Read the model definition and answer for the solid it produces. Units are mm, in the model's axes. Face numbers are marked on the shaded views. A direction names the side the tool comes from. Give positions to 0.01 mm unless a question says otherwise; leave off trailing zeros. Write each loop counter-clockwise with the first axis right and the second up, starting at its lowest first coordinate (ties: lowest second). Pieces come first, ordered by that corner, then holes. Notation, with made-up numbers: (-13.75, 83.5) - (0.25, 83.5) arc R33 ccw to (0.25, 117.5) - close; hole circle Ø3 at (-20.5, 21.25). An arc over 180 degrees is marked (long way). Answer as CSV lines item,"result".
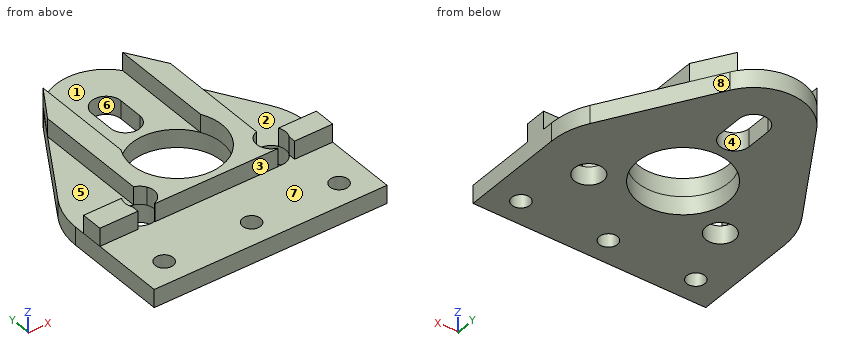
```python
from build123d import *

# Parameters (mm, degrees)
F0_R     = 2.5
F0_R_2   = 4
F0_R_3   = 12.5
F1_DEPTH = 5
F3_DEPTH = 5


# Not quite as in the source:
# - after a boolean that leaves OpenCascade's solid faulty, fix() repairs it


with BuildPart() as f1:
    # F0 (on Top) → F1 (new body)
    with BuildSketch(Plane.XY):
        with BuildLine():
            Line((-32.1865334795, -5.601415029), (-32.1865334795, -34.5))
            Line((-32.1865334795, -34.5), (32.1865334795, -34.5))
            Line((32.1865334795, -34.5), (32.1865334795, -5.601415029))
            ThreePointArc((32.1865334795, -5.601415029), (31.4454600423, -0.2075529944), (29.2771587146, 4.7865842524))
            Line((29.2771587146, 4.7865842524), (11.9634376646, 33.271599497))
            ThreePointArc((11.9634376646, 33.271599497), (0, 40), (-11.9634376646, 33.271599497))
            Line((-11.9634376646, 33.271599497), (-29.2771587146, 4.7865842524))
            ThreePointArc((-29.2771587146, 4.7865842524), (-31.4454600423, -0.2075529944), (-32.1865334795, -5.601415029))
        make_face()
        with Locations((-24.1865334795, -27.5)):
            Circle(F0_R, mode=Mode.SUBTRACT)
        with Locations((-18.1865334795, -10.5)):
            Circle(F0_R_2, mode=Mode.SUBTRACT)
        with Locations((0, -27.5)):
            Circle(F0_R, mode=Mode.SUBTRACT)
        with Locations((24.1865334795, -27.5)):
            Circle(F0_R, mode=Mode.SUBTRACT)
        Circle(F0_R_3, mode=Mode.SUBTRACT)
        with Locations((18.1865334795, -10.5)):
            Circle(F0_R_2, mode=Mode.SUBTRACT)
        with BuildLine():
            Line((-4, 21), (-4, 26))
            ThreePointArc((-4, 26), (0, 30), (4, 26))
            Line((4, 26), (4, 21))
            Line((4, 21), (4, 19))
            ThreePointArc((4, 19), (0, 15), (-4, 19))
            Line((-4, 19), (-4, 21))
        make_face(mode=Mode.SUBTRACT)
    extrude(amount=F1_DEPTH)

    # F2 (on face) → F3 (join)
    with BuildSketch(Plane.XY.offset(5)):
        with BuildLine():
            Line((-32.1865334795, -8.5), (-32.1865334795, -14.5))
            Line((-32.1865334795, -14.5), (-21.6506350946, -14.5))
            Line((-21.6506350946, -14.5), (-21.6506350946, -12.5))
            ThreePointArc((-21.6506350946, -12.5), (-22.1865334795, -10.5), (-21.6506350946, -8.5))
            Line((-21.6506350946, -8.5), (-32.1865334795, -8.5))
        make_face()
        with BuildLine():
            Line((21.6506350946, -14.5), (32.1865334795, -14.5))
            Line((32.1865334795, -14.5), (32.1865334795, -8.5))
            Line((32.1865334795, -8.5), (21.6506350946, -8.5))
            ThreePointArc((21.6506350946, -8.5), (22.1865334795, -10.5), (21.6506350946, -12.5))
            Line((21.6506350946, -12.5), (21.6506350946, -14.5))
        make_face()
        with BuildLine():
            ThreePointArc((17, -14.3199657462), (14.4616036791, -11.9577029816), (14.7224318643, -8.5))
            ThreePointArc((14.7224318643, -8.5), (15.6895011358, -7.3751272866), (17, -6.6800342538))
            Line((17, -6.6800342538), (17, 24.9853071114))
            Line((17, 24.9853071114), (11, 34.6602540378))
            Line((11, 34.6602540378), (11, 5.9371710435))
            ThreePointArc((11, 5.9371710435), (0, -12.5), (-11, 5.9371710435))
            Line((-11, 5.9371710435), (-11, 34.6602540378))
            Line((-11, 34.6602540378), (-17, 24.9853071114))
            Line((-17, 24.9853071114), (-17, -6.6800342538))
            ThreePointArc((-17, -6.6800342538), (-15.6895011358, -7.3751272866), (-14.7224318643, -8.5))
            ThreePointArc((-14.7224318643, -8.5), (-14.4616036791, -11.9577029816), (-17, -14.3199657462))
            Line((-17, -14.3199657462), (-17, -14.5))
            Line((-17, -14.5), (17, -14.5))
            Line((17, -14.5), (17, -14.3199657462))
        make_face()
    extrude(amount=F3_DEPTH)

    add(f1.part.fix(), mode=Mode.REPLACE)


solid = f1.part
```
(1) A cutting plane is placed at D-D (y = 18). Write down the section's boundary in (x, z), and give its area (3 significant figures).
Worked out:
outline,"(-21.25, 0) - (-3.87, 0) - (-3.87, 5) - (-11, 5) - (-11, 10) - (-17, 10) - (-17, 5) - (-21.25, 5) - close; (3.87, 0) - (21.25, 0) - (21.25, 5) - (17, 5) - (17, 10) - (11, 10) - (11, 5) - (3.87, 5) - close"
area,"234 mm^2"
(2) A cutting plane is placed at A-A (x = 0). Write down the section's boundary in (y, z), and give its area (4 significant figures).
Worked out:
outline,"(-34.5, 0) - (-30, 0) - (-30, 5) - (-34.5, 5) - close; (-25, 0) - (-12.5, 0) - (-12.5, 10) - (-14.5, 10) - (-14.5, 5) - (-25, 5) - close; (12.5, 0) - (15, 0) - (15, 5) - (12.5, 5) - close; (30, 0) - (40, 0) - (40, 5) - (30, 5) - close"
area,"157.5 mm^2"
(3) Each of these flat-tipped pins is pushed along its axis until it touches: P1, Ø6, axis at x = -24.5, z = 8.5, coming from the -Y side; P2, Ø2.5, axis at y = 2.5, z = 6.5, coming from the -X side; P3, Ø5.5, axis at y = 21.5, z = 3, coming from the -X side; P4, Ø1.8, axis at x = -15.5, y = 30, coming from the +Z side. Where does it stop, or does it pass through?
Worked out:
P1,"stops at y = -14.5"
P2,"stops at x = -17"
P3,"stops at x = -20.79"
P4,"passes through"
(4) The mould has two halves that part along Y. Classify the marked faces 6, 7 and 8: +Y half, -Y half, draft (parallel to the pull), parting line (faces both ways), or undercut.
Worked out:
face 6,"undercut"
face 7,"draft"
face 8,"+Y half"
(5) A cutting plane is placed at C-C (z = 3). Write down the section's boundary in (x, y).
Worked out:
outline,"(-32.19, -34.5) - (32.19, -34.5) - (32.19, -5.6) arc R20 ccw to (29.28, 4.79) - (11.96, 33.27) arc R14 ccw to (-11.96, 33.27) - (-29.28, 4.79) arc R20 ccw to (-32.19, -5.6) - close; hole circle Ø5 at (-24.19, -27.5); hole circle Ø8 at (-18.19, -10.5); hole circle Ø25 at (0, 0); hole (-4, 19) arc R4 ccw to (4, 19) - (4, 26) arc R4 ccw to (-4, 26) - close; hole circle Ø5 at (0, -27.5); hole circle Ø8 at (18.19, -10.5); hole circle Ø5 at (24.19, -27.5)"
(6) For the marked faces 1, 2, 3, 4 and 5, determine the directions among +Z, -Z, +X, -X, +Y, -Y from which every point of the face is accessible in a straight line to the end or side of a thin tool.
Worked out:
face 1,"+Z, +Y"
face 2,"+Z, +X, +Y"
face 3,"+Z, +X, -X, -Y"
face 4,"+Z, -Z"
face 5,"+Z, -X, +Y"
(7) Find the intervals of material crossed by L1, parallel to Y at x = 0, z = 4; L2, parallel to X at y = 21, z = 6; L3, parallel to X at y = -0.5, z = 6.25, in increasing order.
Worked out:
L1,"y = -34.5 to -30, -25 to -12.5, 12.5 to 15, 30 to 40"
L2,"x = -17 to -11, 11 to 17"
L3,"x = -17 to -12.49, 12.49 to 17"
(8) A cutting plane is placed at B-B (z = 6.5). Write down the section's boundary in (x, y).
Worked out:
outline,"(-32.19, -14.5) - (-21.65, -14.5) - (-21.65, -12.5) arc R4 cw to (-21.65, -8.5) - (-32.19, -8.5) - close; (-17, -14.5) - (17, -14.5) - (17, -14.32) arc R4 cw to (17, -6.68) - (17, 24.99) - (11, 34.66) - (11, 5.94) arc R12.5 cw (long way) to (-11, 5.94) - (-11, 34.66) - (-17, 24.99) - (-17, -6.68) arc R4 cw to (-17, -14.32) - close; (21.65, -14.5) - (32.19, -14.5) - (32.19, -8.5) - (21.65, -8.5) arc R4 cw to (21.65, -12.5) - close"
